from build123d import *

# Parameters (mm, degrees)
SKETCH2_R           = 7.62
BOSS_EXTRUDE1_DEPTH = 1.27
BOSS_EXTRUDE2_DEPTH = 7.62
SKETCH4_R           = 5.715
BOSS_EXTRUDE3_DEPTH = 1.27
SKETCH5_R           = 6.35
BOSS_EXTRUDE4_DEPTH = 1.27
FILLET1_R           = 0.254
SKETCH6_R           = 2
CUT_EXTRUDE1_DEPTH  = 11.43


with BuildPart() as part:
    # Sketch2 → Boss-Extrude1 (new body)
    with BuildSketch(Plane(origin=(0, 0, 0), x_dir=(0, 0, -1), z_dir=(1, 0, 0))):
        Circle(SKETCH2_R)
    extrude(amount=-BOSS_EXTRUDE1_DEPTH)

    # Sketch3 → Boss-Extrude2 (add)
    with BuildSketch(Plane(origin=(0, 0, 0), x_dir=(0, 0, -1), z_dir=(1, 0, 0))):
        Polygon((-3.666174209, 6.35), (-7.332348419, 0), (-3.666174209, -6.35), (3.666174209, -6.35), (7.332348419, 0), (3.666174209, 6.35), align=None)
    extrude(amount=BOSS_EXTRUDE2_DEPTH)

    # Sketch4 → Boss-Extrude3 (add)
    with BuildSketch(Plane(origin=(7.62, 0, 0), x_dir=(0, 0, -1), z_dir=(1, 0, 0))):
        Circle(SKETCH4_R)
    extrude(amount=BOSS_EXTRUDE3_DEPTH)

    # Sketch5 → Boss-Extrude4 (add)
    with BuildSketch(Plane(origin=(8.89, 0, 0), x_dir=(0, 0, -1), z_dir=(1, 0, 0))):
        Circle(SKETCH5_R)
    extrude(amount=BOSS_EXTRUDE4_DEPTH)

    # Fillet1
    fillet1_edges = [part.edges().sort_by_distance(p)[0] for p in [
        (8.89, 0, 5.715),
        (8.89, 0, 6.35),
    ]]
    fillet(fillet1_edges, radius=FILLET1_R)

    # Sketch6 → Cut-Extrude1 (cut)
    with BuildSketch(Plane(origin=(10.16, 0, 0), x_dir=(0, 0, -1), z_dir=(1, 0, 0))):
        Circle(SKETCH6_R)
    extrude(amount=-CUT_EXTRUDE1_DEPTH, mode=Mode.SUBTRACT)


solid = part.part
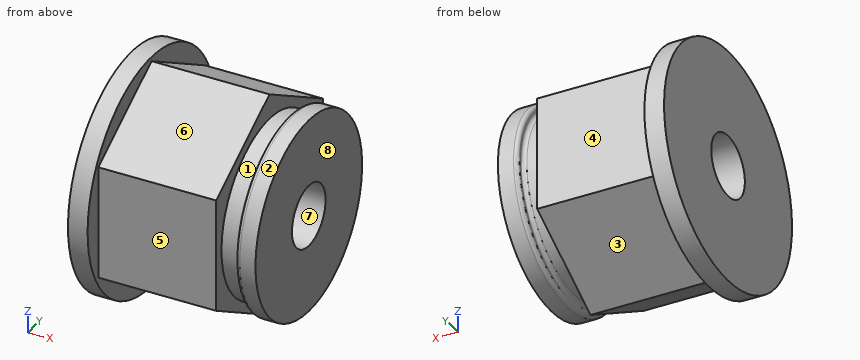
Could you check a few things on this model? Use its own coordinates, in mm. Face numbers are marked on the shaded views. A direction names the side the tool comes from. Give positions to 0.01 mm unless a question says otherwise; leave off trailing zeros. Write each loop counter-clockwise with the first axis right and the second up, starting at its lowest first coordinate (ties: lowest second). Pieces come first, ordered by that corner, then holes. Notation, with made-up numbers: (-23.75, 37.5) -> (30.25, 37.5) arc R25 ccw to (30.25, 52.5) -> close; hole circle Ø11 at (-29.5, 26). An arc over 180 degrees is marked (long way). Answer as a JSON object with one key per item and string values.
Q1. We'd pull the mould along Z, two halves only. Please class the marked faces 6, 7 and 8: released by +Z, released by -Z, zero draft, split by the parting line, or undercut.
Taken from the geometry:
{"face 6": "released by +Z", "face 7": "undercut", "face 8": "zero draft"}
Q2. Will these pins go through, and if not, where does the flat tip stop? pin 1 Ø4 at (x, y) = (9, 3.5) entering from -Z; pin 2 Ø1.5 at (x, z) = (1, -1.5) entering from +Y; pin 3 Ø3.5 at (y, z) = (-1.5, -0.5) entering from -X.
Taken from the geometry:
{"pin 1": "stops at z = -6.17", "pin 2": "stops at y = 6.35", "pin 3": "stops at x = -1.27"}
Q3. Suppose I cut it at B-B on z = 0. Write out the boundary of the cut face in (x, y) (3 decimals).
Taken from the geometry:
{"outline": "(-1.27, -7.62) -> (0, -7.62) -> (0, -6.35) -> (7.62, -6.35) -> (7.62, -5.715) -> (8.636, -5.715) arc R0.254 cw to (8.89, -5.969) -> (8.89, -6.096) arc R0.254 ccw to (9.144, -6.35) -> (10.16, -6.35) -> (10.16, -2) -> (-1.27, -2) -> close; (-1.27, 2) -> (10.16, 2) -> (10.16, 6.35) -> (9.144, 6.35) arc R0.254 ccw to (8.89, 6.096) -> (8.89, 5.969) arc R0.254 cw to (8.636, 5.715) -> (7.62, 5.715) -> (7.62, 6.35) -> (0, 6.35) -> (0, 7.62) -> (-1.27, 7.62) -> close"}
Q4. Suppose I cut it at A-A on x = 0.25. Write out the boundary of the cut face in (y, z).
Taken from the geometry:
{"outline": "(-6.35, -3.67) -> (0, -7.33) -> (6.35, -3.67) -> (6.35, 3.67) -> (0, 7.33) -> (-6.35, 3.67) -> close; hole circle Ø4 at (0, 0)"}
Q5. Please list where these lines run through material, in increasing order: L1, parallel to X at y = 2.25, z = 5.5; L2, parallel to Y at x = 2.5, z = 0; L3, parallel to X at y = -4, z = -5.25.
Taken from the geometry:
{"L1": "x = -1.27 to 7.62, 8.89 to 10.16", "L2": "y = -6.35 to -2, 2 to 6.35", "L3": "x = -1.27 to 0"}
Q6. Which directions (+Z, -Z, +X, -X, +Y, -Y) give clear straight access to the entire face, cutting with the end or side of a thin tool? Please do the marked faces 1, 2, 3, 4 and 5.
Taken from the geometry:
{"face 1": "none", "face 2": "+X", "face 3": "-Z, +X, +Y", "face 4": "+Z, -Z, +X, +Y", "face 5": "+Z, -Z, +X, -Y"}
